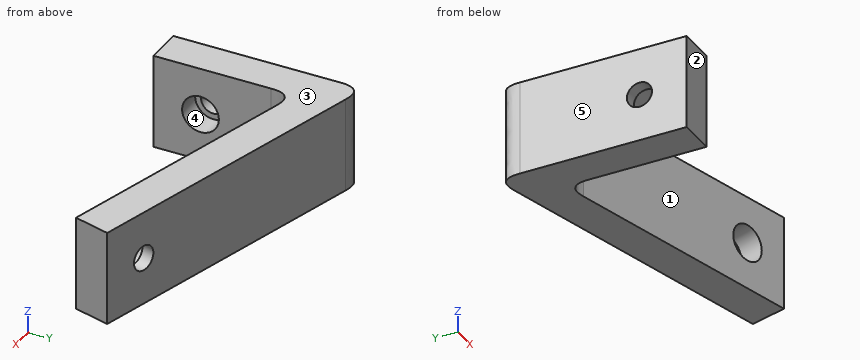
from build123d import *

# Parameters (mm, degrees)
BOSS_EXTRUDE1_DEPTH         = 25.4
F_1_4_CLEARANCE_HOLE1_D     = 6.7564
F_1_4_CLEARANCE_HOLE1_DEPTH = 10.16
F_1_4_CLEARANCE_HOLE1_TIP   = 2.029827343
F_1_4_CLEARANCE_HOLE2_D     = 6.7564
F_1_4_CLEARANCE_HOLE2_DEPTH = 10.16
F_1_4_CLEARANCE_HOLE2_TIP   = 2.029827343
SKETCH8_R                   = 4.953
CUT_EXTRUDE1_DEPTH          = 6.604
SKETCH9_R                   = 4.953
CUT_EXTRUDE2_DEPTH          = 6.604


with BuildPart() as part:
    # Sketch1 → Boss-Extrude1 (new body)
    with BuildSketch(Plane.XY):
        Polygon((10.16, 0), (0, 0), (0, 51.340769788), (86.393149461, 28.191795158), (83.763547963, 18.377988763), (10.16, 38.1), align=None)
    extrude(amount=BOSS_EXTRUDE1_DEPTH)

    # 1/4 Clearance Hole1
    with Locations(Plane.ZY):
        with Locations((12.7, 12.7)):
            Hole(F_1_4_CLEARANCE_HOLE1_D / 2, depth=F_1_4_CLEARANCE_HOLE1_DEPTH)
            with Locations((0, 0, -(F_1_4_CLEARANCE_HOLE1_DEPTH + F_1_4_CLEARANCE_HOLE1_TIP / 2))):  # 118° drill point
                Cone(0, F_1_4_CLEARANCE_HOLE1_D / 2, F_1_4_CLEARANCE_HOLE1_TIP, mode=Mode.SUBTRACT)

    # 1/4 Clearance Hole2
    with Locations(Plane(origin=(12.835192447, 47.901590337, 0), x_dir=(0.9659258262890674, -0.2588190451025242, 0), z_dir=(0.2588190451025242, 0.9659258262890674, 0))):
        with Locations((63.452800777, -12.7)):
            Hole(F_1_4_CLEARANCE_HOLE2_D / 2, depth=F_1_4_CLEARANCE_HOLE2_DEPTH)
            with Locations((0, 0, -(F_1_4_CLEARANCE_HOLE2_DEPTH + F_1_4_CLEARANCE_HOLE2_TIP / 2))):  # 118° drill point
                Cone(0, F_1_4_CLEARANCE_HOLE2_D / 2, F_1_4_CLEARANCE_HOLE2_TIP, mode=Mode.SUBTRACT)

    # Fillet1
    # a fillet whose section is not a circle: 5.08 mm, written as the material it adds along each edge (its section moved 0.00015 mm through the faces so that the kernel can cut it)
    with BuildSketch(Plane(origin=(10.16, 38.1, 0), x_dir=(0.9659316901800618, -0.25879715977168133, 0), z_dir=(0, 0, 1))) as fillet1_piece_1:
        with BuildLine():
            add(Edge.make_bspline([(6.620384896, 0), (5.560159502, 2.4022e-05), (4.499934108, 4.8044e-05), (2.201778974, -0.538520049), (1.089942696, -1.987425322), (1.164425276, -4.346667776), (1.438808597, -5.370773083), (1.713191917, -6.39487839)], knots=[0, 0, 0, 0, 0, 0, 0.5, 0.5, 1, 1, 1, 1, 1, 1], degree=5))
            Line((1.713191917, -6.39487839), (1.615053258, -6.421172181))
            ThreePointArc((1.615053258, -6.421172181), (0.758529744, -3.223713577), (-0.09813866, -0.026293791))
            Line((-0.09813866, -0.026293791), (2.302e-06, 0.1016))
            ThreePointArc((2.302e-06, 0.1016), (3.310194748, 0.101525), (6.620387198, 0.1016))
            Line((6.620387198, 0.1016), (6.620384896, 0))
        make_face()
    extrude(amount=25.4)
    # a fillet whose section is not a circle: 5.08 mm, written as the material it takes off along each edge (its section moved 0.00015 mm through the faces so that the kernel can cut it)
    with BuildSketch(Plane(origin=(0, 51.340769788, -16.550962239), x_dir=(-2.2657292946318672e-05, -0.9999999997433235, 0), z_dir=(0, 0, 1))) as fillet1_2_piece_1:
        with BuildLine():
            add(Edge.make_bspline([(6.620384896, 0), (5.560159502, -2.4022e-05), (4.499934108, -4.8044e-05), (2.201778974, 0.538520049), (1.089942696, 1.987425322), (1.164425276, 4.346667776), (1.438808597, 5.370773083), (1.713191917, 6.39487839)], knots=[0, 0, 0, 0, 0, 0, 0.5, 0.5, 1, 1, 1, 1, 1, 1], degree=5))
            Line((1.713191917, 6.39487839), (1.615053258, 6.421172181))
            ThreePointArc((1.615053258, 6.421172181), (0.758529744, 3.223713577), (-0.09813866, 0.026293791))
            Line((-0.09813866, 0.026293791), (2.302e-06, -0.1016))
            ThreePointArc((2.302e-06, -0.1016), (3.310194748, -0.101525), (6.620387198, -0.1016))
            Line((6.620387198, -0.1016), (6.620384896, 0))
        make_face()
    extrude(amount=58.501924479, mode=Mode.SUBTRACT)

    # Sketch8 → Cut-Extrude1 (cut)
    with BuildSketch(Plane(origin=(10.205590949, 38.087783942, 0), x_dir=(0.9659258262890673, -0.2588190451025246, 0), z_dir=(-0.2588190451025246, -0.9659258262890674, 0))):
        with Locations((63.452800777, 12.7)):
            Circle(SKETCH8_R)
    extrude(amount=-CUT_EXTRUDE1_DEPTH, mode=Mode.SUBTRACT)

    # Sketch9 → Cut-Extrude2 (cut)
    with BuildSketch(Plane(origin=(10.16, 0, 0), x_dir=(0, 0, -1), z_dir=(1, 0, 0))):
        with Locations(Location((-12.7, 12.7, 0), (0, 0, 90))):
            Circle(SKETCH9_R)
    extrude(amount=-CUT_EXTRUDE2_DEPTH, mode=Mode.SUBTRACT)


solid = part.part
Verification items for the finished model (mm, model axes). Face numbers are marked on the shaded views. A direction names the side the tool comes from. Give positions to 0.01 mm unless a question says otherwise; leave off trailing zeros. Order: outer loops, then holes, each group sorted by start corner. A loop starts at its lowest first (then second) coordinate and runs counter-clockwise, first axis right, second up. Notation, with made-up numbers: M 4,0.25 L 8,0.25 A17 ccw 8,25.25 Z; hole C 62,45.25 d4. An arc over 180 degrees is marked long. Use one line per item in the form item = value. Start each with the question number.
Q1. Scan lines: line 1 along Z through (x, y) = (6, 12); line 2 along Y through (x, z) = (1.25, 12.7); line 3 along Y through (x, z) = (0.9, 12.7). Record each from-to range of solid material in increasing order. Write a range as [from, to].
Q2. Section check C-C (y = 3). Enter the section's corners in (x, z), then the cut area to 3 significant figures.
Q3. Section check A-A (y = 12.7). Enter the section's corners in (x, z), then the cut area to 3 significant figures.
Q4. Access from +Z, -Z, +X, -X, +Y, -Y to the whole of each face (thin tool, end or side, straight path). Record for the marked faces 1 and 2.
Q5. Mould release check, pull along Z, two halves, no side actions. Record for the marked faces 3, 4 and 5: +Z half, -Z half, draft (parallel to the pull), parting line (faces both ways), or undercut.
Q6. Section check B-B (z = 12.7). Count the separate pieces of the cut face and the enclosed holes in it, then the cut area to 3 significant figures.
Q7. Section check D-D (x = 24). Enter the section's corners in (y, z), then the cut area to 3 significant figures.
Q8. Go/stop test with flat-tipped pins: pin 1 Ø10 at (x, y) = (56, 42.5) entering from -Z; pin 2 Ø7.5 at (y, z) = (15.5, 13) entering from +X; pin 3 Ø8 at (y, z) = (12, 11) entering from +X; pin 4 Ø8 at (y, z) = (31.5, 12.5) entering from +X. Record where each tip stops, or that it passes through.
Evaluation:
q1.line_1 = [0, 7.8], [17.6, 25.4]
q1.line_2 = [0, 9.32], [16.08, 49.19]
q1.line_3 = [0, 9.32], [16.08, 48.79]
q2.outline = M 0,0 L 10.16,0 L 10.16,25.4 L 0,25.4 Z
q2.area = 258 mm2
q3.outline = M 0,0 L 10.16,0 L 10.16,7.75 L 3.56,7.75 L 3.56,9.32 L 0,9.32 Z; M 0,16.08 L 3.56,16.08 L 3.56,17.65 L 10.16,17.65 L 10.16,25.4 L 0,25.4 Z
q3.area = 169 mm2
q4.face_1 = +Z, -Z, -Y
q4.face_2 = +Z, -Z, +X, -X, -Y
q5.face_3 = +Z half
q5.face_4 = undercut
q5.face_5 = draft
q6.separate_pieces = 3
q6.enclosed_holes = 0
q6.area = 1,120 mm2
q7.outline = M 34.39,0 L 44.91,0 L 44.91,25.4 L 34.39,25.4 Z
q7.area = 267 mm2
q8.pin_1 = through
q8.pin_2 = 84
q8.pin_3 = 10.16
q8.pin_4 = 86.39
